Check sheet for the modelled part. Datum: model origin and axes. Units: mm. Face numbers are marked on the shaded views. A direction names the side the tool comes from. Coordinates: 2 decimals unless noted, no trailing zeros. Loops run counter-clockwise (first coordinate to the right, second up) from the corner with the lowest first, then second, coordinate; pieces in that order, holes last. Notation, with made-up numbers: (68.5, 4.25) - (120.5, 4.25) arc R19 cw to (120.5, 14.25) - close; hole circle Ø5 at (1, -5). An arc over 180 degrees is marked (long way). Use a Markdown table: item, result. Add a question column.
1) Tool access check on the marked faces 1 and 2. Record the directions out of +Z, -Z, +X, -X, +Y, -Y that give a thin tool (end or side, any length) a straight path to the whole face; none if there is none.
2) Thickness scan on line 1 (X direction, y = 1, z = 0); line 2 (Z direction, x = 0, y = 159). Record the ranges inside material, lowest first.
3) Draft check along X on the marked faces 3, 4 and 5. Enter one of: pulls with the +X half, pulls with the -X half, needs draft (parallel to the pull), parting line crosses it, or undercut.
4) Go/stop test with flat-tipped pins: P1, Ø1.5, axis at y = 110.5, z = -21.5, coming from the -X side; P2, Ø1, axis at x = -46, z = -36, coming from the +Y side; P3, Ø21, axis at x = -4.5, z = 4.5, coming from the +Y side; P4, Ø8, axis at y = 101.5, z = 7.5, coming from the +X side. Record where each tip stops, or that it passes through.
5) Sectioned sample at B-B, the plane x = 0. Enter the section's corners in (y, z), then the cut area to 3 significant figures.
6) Sectioned sample at D-D, the plane y = 100. Enter the section's corners in (x, z), then the cut area to 3 significant figures.
7) Sectioned sample at C-C, the plane y = 158.5. Enter the section's corners in (x, z), then the cut area to 3 significant figures.
8) Sectioned sample at A-A, the plane z = 0. Enter the section's corners in (x, y), then the cut area to 3 significant figures.
Autodesk Inventor part; units mm, degrees
ref_plane "YZ Plane" through (0, 0, 0) normal (1, 0, 0) x (0, 1, 0)
ref_plane "XZ Plane" through (0, 0, 0) normal (0, 1, 0) x (-1, 0, 0)
ref_plane "XY Plane" through (0, 0, 0) normal (0, 0, 1) x (1, 0, 0)
sketch "FV.sec" plane through (0, 0, 0) normal (0, 0, 1) x (1, 0, 0)
  line L0 (25, 185) -> (35, 185)
  line L1 (35, 185) -> (35, 145)
  line L2 (25, 185) -> (25, 129.6172)
  line L3 (50, 20) -> (70, 20)
  line L4 (70, 20) -> (70, 0)
  line L5 (0, 0) -> (0, 185)
  line L6 (35, 145) -> (35.2904, 145)
  line L7 (33.3087, 142.7305) -> (50, 20)
  line L8 (70, 0) -> (50, 0)
  line L9 (50, 0) -> (50, 3)
  line L10 (50, 3) -> (42.2199, 3)
  line L11 (42.2199, 3) -> (25, 129.6172)
  arc A0 (35.2904, 145) -> (33.3087, 142.7305) centre (35.2904, 143) ccw
  point P0 (33, 145)
  dimension "d9" = 40
  dimension "d11" = 185
  dimension "d12" = 20
  dimension "d16" = 3
  dimension "d17" = 10
  dimension "d18" = 66
  dimension "d21" = 100
  dimension "d22" = 10
  dimension "d23" = 100
  dimension "d24" = 20
  dimension "d28" = 2
revolve "Revolution1" add sketch "FV.sec" angle 360 about axis through (0, 0, 0) along (0, 1, 0)
fillet "Fillet1" radius 8 1 edges at (-50, 20, 0)
properties material "Iron, Cast"
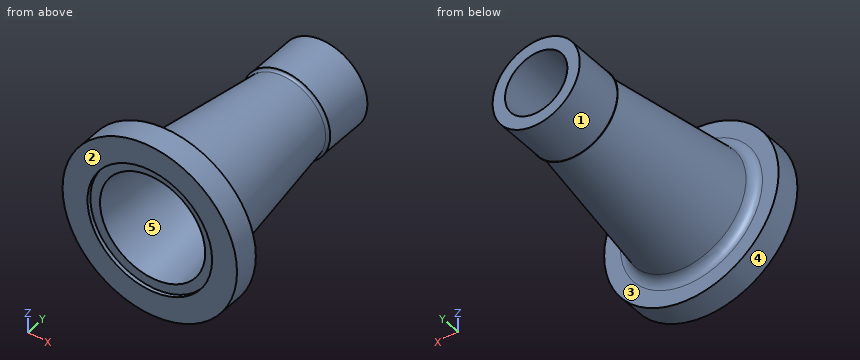
Solved:
| question | item | result |
|---|---|---|
| 1 | face 1 | +Y |
| 1 | face 2 | +Z, -Z, +X, -X, -Y |
| 2 | line 1 | x = -70 to -50, 50 to 70 |
| 2 | line 2 | z = -35 to -25, 25 to 35 |
| 3 | face 3 | needs draft |
| 3 | face 4 | parting line crosses it |
| 3 | face 5 | undercut |
| 4 | P1 | stops at x = -31.48 |
| 4 | P2 | stops at y = 20 |
| 4 | P3 | passes through |
| 4 | P4 | stops at x = 39.02 |
| 5 | outline | (0, -70) - (20, -70) - (20, -56.99) arc R8 cw to (26.92, -49.06) - (142.73, -33.31) arc R2 cw to (145, -35.29) - (145, -35) - (185, -35) - (185, -25) - (129.62, -25) - (3, -42.22) - (3, -50) - (0, -50) - close; (0, 50) - (3, 50) - (3, 42.22) - (129.62, 25) - (185, 25) - (185, 35) - (145, 35) - (145, 35.29) arc R2 cw to (142.73, 33.31) - (26.92, 49.06) arc R8 cw to (20, 56.99) - (20, 70) - (0, 70) - close |
| 5 | area | 4,420 mm2 |
| 6 | outline | circle Ø78.24 at (0, 0); hole circle Ø58.06 at (0, 0) |
| 6 | area | 2,160 mm2 |
| 7 | outline | circle Ø70 at (0, 0); hole circle Ø50 at (0, 0) |
| 7 | area | 1,880 mm2 |
| 8 | outline | (-70, 0) - (-50, 0) - (-50, 3) - (-42.22, 3) - (-25, 129.62) - (-25, 185) - (-35, 185) - (-35, 145) - (-35.29, 145) arc R2 cw to (-33.31, 142.73) - (-49.06, 26.92) arc R8 cw to (-56.99, 20) - (-70, 20) - close; (25, 129.62) - (42.22, 3) - (50, 3) - (50, 0) - (70, 0) - (70, 20) - (56.99, 20) arc R8 cw to (49.06, 26.92) - (33.31, 142.73) arc R2 cw to (35.29, 145) - (35, 145) - (35, 185) - (25, 185) - close |
| 8 | area | 4,420 mm2 |
